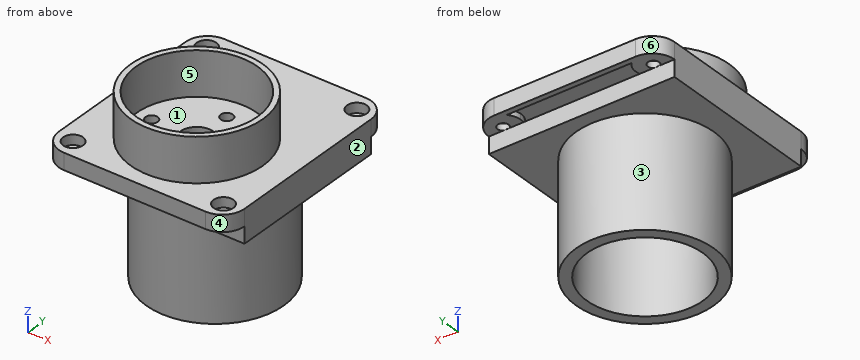
from build123d import *

# Parameters (mm, degrees)
SZKIC1_R                    = 3
SZKIC1_R_2                  = 1.1
SZKIC1_R_3                  = 1
DODANIE_WYCI_GNI_CIE1_DEPTH = 3
SZKIC2_R                    = 12
SZKIC2_R_2                  = 11
DODANIE_WYCI_GNI_CIE2_DEPTH = 8
SZKIC3_R                    = 1.1
SZKIC3_R_2                  = 3
WYTNIJ_WYCI_GNI_CIE1_DEPTH  = 1
SZKIC4_R                    = 1.8
WYTNIJ_WYCI_GNI_CIE2_DEPTH  = 1.8
ZAOKR_GLENIE1_R             = 4
SKETCH1_W                   = 33.7
SKETCH1_H                   = 30
BOSS_EXTRUDE1_DEPTH         = 3
SKETCH2_R                   = 12.5
SKETCH2_R_2                 = 10.5
BOSS_EXTRUDE2_DEPTH         = 20


with BuildPart() as part:
    # Szkic1 → Dodanie-wyciągnięcie1 (new body)
    with BuildSketch(Plane.XY):
        Polygon((-16.85, 0), (-16.85, -14.7), (0, -14.7), (16.85, -14.7), (16.85, 23.3), (-16.85, 23.3), align=None)
        Circle(SZKIC1_R, mode=Mode.SUBTRACT)
        with Locations((-8.2, 0)):
            Circle(SZKIC1_R_2, mode=Mode.SUBTRACT)
        with Locations((8.2, 0)):
            Circle(SZKIC1_R_2, mode=Mode.SUBTRACT)
        with Locations((0, 7.1)):
            Circle(SZKIC1_R_2, mode=Mode.SUBTRACT)
        with Locations((0, -7.1)):
            Circle(SZKIC1_R_2, mode=Mode.SUBTRACT)
        with Locations((-13.65, 20.1)):
            Circle(SZKIC1_R_3, mode=Mode.SUBTRACT)
        with Locations((13.65, 20.1)):
            Circle(SZKIC1_R_3, mode=Mode.SUBTRACT)
        with Locations((13.65, -11.5)):
            Circle(SZKIC1_R_3, mode=Mode.SUBTRACT)
        with Locations((-13.65, -11.5)):
            Circle(SZKIC1_R_3, mode=Mode.SUBTRACT)
    extrude(amount=DODANIE_WYCI_GNI_CIE1_DEPTH)

    # Szkic2 → Dodanie-wyciągnięcie2 (add)
    with BuildSketch(Plane.XY.offset(3)):
        Circle(SZKIC2_R)
        Circle(SZKIC2_R_2, mode=Mode.SUBTRACT)
    extrude(amount=DODANIE_WYCI_GNI_CIE2_DEPTH)

    # Szkic3 → Wytnij-wyciągnięcie1 (cut)
    with BuildSketch(Plane(origin=(0, 0, 0), x_dir=(-1, 0, 0), z_dir=(0, 0, -1))):
        with BuildLine():
            Line((11.326209992, 22.3), (-11.326209992, 22.3))
            ThreePointArc((-11.326209992, 22.3), (-10.67711184, 21.284033778), (-10.45, 20.1))
            ThreePointArc((-10.45, 20.1), (-12.385088936, 17.160612309), (-15.85, 17.776209992))
            Line((-15.85, 17.776209992), (-15.85, -9.176209992))
            ThreePointArc((-15.85, -9.176209992), (-12.385088936, -8.560612309), (-10.45, -11.5))
            ThreePointArc((-10.45, -11.5), (-10.67711184, -12.684033778), (-11.326209992, -13.7))
            Line((-11.326209992, -13.7), (11.326209992, -13.7))
            ThreePointArc((11.326209992, -13.7), (11.3872583, -9.2372583), (15.85, -9.176209992))
            Line((15.85, -9.176209992), (15.85, 17.776209992))
            ThreePointArc((15.85, 17.776209992), (11.3872583, 17.8372583), (11.326209992, 22.3))
        make_face()
        with Locations((-8.2, 0)):
            Circle(SZKIC3_R, mode=Mode.SUBTRACT)
        with Locations((0, -7.1)):
            Circle(SZKIC3_R, mode=Mode.SUBTRACT)
        Circle(SZKIC3_R_2, mode=Mode.SUBTRACT)
        with Locations((8.2, 0)):
            Circle(SZKIC3_R, mode=Mode.SUBTRACT)
        with Locations((0, 7.1)):
            Circle(SZKIC3_R, mode=Mode.SUBTRACT)
    extrude(amount=-WYTNIJ_WYCI_GNI_CIE1_DEPTH, mode=Mode.SUBTRACT)

    # Szkic4 → Wytnij-wyciągnięcie2 (cut)
    with BuildSketch(Plane.XY.offset(3)):
        with Locations((-13.65, 20.1)):
            Circle(SZKIC4_R)
        with Locations((13.65, 20.1)):
            Circle(SZKIC4_R)
        with Locations((13.65, -11.5)):
            Circle(SZKIC4_R)
        with Locations((-13.65, -11.5)):
            Circle(SZKIC4_R)
    extrude(amount=-WYTNIJ_WYCI_GNI_CIE2_DEPTH, mode=Mode.SUBTRACT)

    # Zaokrąglenie1
    zaokr_glenie1_edges = [part.edges().sort_by_distance(p)[0] for p in [
        (-16.85, 23.3, 1.5),
        (16.85, 23.3, 1.5),
        (16.85, -14.7, 1.5),
        (-16.85, -14.7, 1.5),
    ]]
    fillet(zaokr_glenie1_edges, radius=ZAOKR_GLENIE1_R)

    # Sketch1 → Boss-Extrude1 (add)
    with BuildSketch(Plane(origin=(0, 0, 0), x_dir=(-1, 0, 0), z_dir=(0, 0, -1))):
        with Locations((0, 4.3)):
            Rectangle(SKETCH1_W, SKETCH1_H)
    extrude(amount=BOSS_EXTRUDE1_DEPTH)

    # Sketch2 → Boss-Extrude2 (add)
    with BuildSketch(Plane(origin=(0, 0, -3), x_dir=(-1, 0, 0), z_dir=(0, 0, -1))):
        with Locations((0, 4.3)):
            Circle(SKETCH2_R)
        with Locations((0, 4.3)):
            Circle(SKETCH2_R_2, mode=Mode.SUBTRACT)
    extrude(amount=BOSS_EXTRUDE2_DEPTH)


solid = part.part
Design review of the part built by this model. Coordinates are the model's own, in mm. Face numbers are marked on the shaded views. A direction names the side the tool comes from. Coordinates: 2 decimals unless noted, no trailing zeros. Write each loop counter-clockwise with the first axis right and the second up, starting at its lowest first coordinate (ties: lowest second). Pieces come first, ordered by that corner, then holes. Notation, with made-up numbers: (8, 42.25) -> (41, 42.25) arc R17 ccw to (41, 64.25) -> close; hole circle Ø2 at (10, 35.25). An arc over 180 degrees is marked (long way). Write each question's results on one line, items separated by ' | '. Start each with the question number.
(1) Take a section at B-B on x = -8.2. Give the number of separate pieces and of enclosed holes in the cut face, and give its area (3 significant figures).
(2) Clearance check with flat-ended pins moving along their axes: P1, Ø4.5, axis at x = -13.65, y = 20.1, coming from the -Z side; P2, Ø2, axis at y = 5.5, z = 7, coming from the +X side; P3, Ø3, axis at x = 0.5, z = -19, coming from the +Y side; P4, Ø1.2, axis at x = 13.65, y = 20.1, coming from the -Z side. State where each tip first meets the part, or that it passes through.
(3) For line 1 along Z through (x, y) = (4.5, 16.5); line 2 along Y through (x, z) = (8.2, 1.6); line 3 along Z through (x, y) = (-7, 9.5), list the stretches that pass through material, from the lowest coordinate up. Write a range as from..to.
(4) Take a section at C-C on y = 4.3. Write out the cut boundary in (x, z), and give its area (3 significant figures).
(5) Take a section at A-A on z = 6.5. Write out the cut boundary in (x, y), and give its area (3 significant figures).
(6) Tool access review of the marked faces 1, 2 and 3: name each direction out of +Z, -Z, +X, -X, +Y, -Y from which nothing blocks a thin tool from reaching the whole face with its end or side.
(7) The part is to be moulded in two halves that separate along Y. For the marked faces 4, 5 and 6, say which applies: pulls with the +Y half, pulls with the -Y half, needs draft (parallel to the pull), parting line crosses it, or undercut.
Results found:
1) separate pieces: 3 | enclosed holes: 0 | area: 302 mm2
2) P1: stops at z = -3 | P2: stops at x = 11.12 | P3: stops at y = 16.8 | P4: passes through
3) line 1: z = -3..0, 1..3 | line 2: y = -14.7..-1.1, 1.1..23.3 | line 3: z = -3..0, 1..11
4) outline: (-16.85, -3) -> (-12.5, -3) -> (-12.5, -23) -> (-10.5, -23) -> (-10.5, -3) -> (10.5, -3) -> (10.5, -23) -> (12.5, -23) -> (12.5, -3) -> (16.85, -3) -> (16.85, 3) -> (11.2, 3) -> (11.2, 11) -> (10.12, 11) -> (10.12, 3) -> (-10.12, 3) -> (-10.12, 11) -> (-11.2, 11) -> (-11.2, 3) -> (-16.85, 3) -> close; hole (-15.85, 0) -> (15.85, 0) -> (15.85, 1) -> (-15.85, 1) -> close | area: 268 mm2
5) outline: circle Ø24 at (0, 0); hole circle Ø22 at (0, 0) | area: 72.3 mm2
6) face 1: +Z | face 2: +Z, -Z, +X, +Y, -Y | face 3: -Z
7) face 4: pulls with the -Y half | face 5: undercut | face 6: pulls with the +Y half
